from build123d import *

# Parameters (mm, degrees)
SKETCH3_R                = 50
SKETCH3_R_2              = 25
BOSS_EXTRUDE1_DEPTH      = 30
BOSS_EXTRUDE1_DEPTH_BACK = 30
SKETCH5_R                = 27.5
BOSS_EXTRUDE2_DEPTH      = 90
SKETCH6_R                = 23.5
CUT_EXTRUDE1_DEPTH       = 35
CHAMFER1_SIZE            = 1
CHAMFER3_SIZE            = 1
CHAMFER5_SIZE            = 1
CHAMFER6_SIZE            = 1
CHAMFER7_SIZE            = 1


with BuildPart() as part:
    # Sketch3 → Boss-Extrude1 (new body, two sides)
    with BuildSketch(Plane.XY) as boss_extrude1_sk:
        Circle(SKETCH3_R)
        Circle(SKETCH3_R_2, mode=Mode.SUBTRACT)
    extrude(amount=BOSS_EXTRUDE1_DEPTH)
    extrude(boss_extrude1_sk.sketch, amount=-BOSS_EXTRUDE1_DEPTH_BACK)

    # Sketch4 → Cut-Revolve5 (revolve, cut)
    with BuildSketch(Plane(origin=(0, 0, 0), x_dir=(0, 0, -1), z_dir=(1, 0, 0))):
        with BuildLine():
            Line((0, 32.5), (0, -32.5))
            ThreePointArc((0, -32.5), (32.5, 0), (0, 32.5))
        make_face()
    revolve(axis=Axis((0, 32.5, 0), (0, -1, 0)), mode=Mode.SUBTRACT)

    # Sketch5 → Boss-Extrude2 (add)
    with BuildSketch(Plane(origin=(125, 0, 0), x_dir=(0, 0, -1), z_dir=(1, 0, 0))):
        Circle(SKETCH5_R)
    extrude(amount=-BOSS_EXTRUDE2_DEPTH)

    # Sketch6 → Cut-Extrude1 (cut)
    with BuildSketch(Plane(origin=(125, 0, 0), x_dir=(0, 0, -1), z_dir=(1, 0, 0))):
        Circle(SKETCH6_R)
    extrude(amount=-CUT_EXTRUDE1_DEPTH, mode=Mode.SUBTRACT)

    # Chamfer1
    chamfer1_edges = [part.edges().sort_by_distance(p)[0] for p in [
        (-50, 0, -30),
    ]]
    chamfer(chamfer1_edges, length=CHAMFER1_SIZE)

    # Chamfer3
    chamfer3_edges = [part.edges().sort_by_distance(p)[0] for p in [
        (-25, 0, -30),
    ]]
    chamfer(chamfer3_edges, length=CHAMFER3_SIZE)

    # Chamfer5
    chamfer5_edges = [part.edges().sort_by_distance(p)[0] for p in [
        (-50, 0, 30),
    ]]
    chamfer(chamfer5_edges, length=CHAMFER5_SIZE)

    # Chamfer6
    chamfer6_edges = [part.edges().sort_by_distance(p)[0] for p in [
        (-25, 0, 30),
    ]]
    chamfer(chamfer6_edges, length=CHAMFER6_SIZE)

    # Chamfer7
    chamfer7_edges = [part.edges().sort_by_distance(p)[0] for p in [
        (125, 0, 27.5),
        (125, 0, 23.5),
    ]]
    chamfer(chamfer7_edges, length=CHAMFER7_SIZE)


solid = part.part
Geometry: final body of the model. Coordinates: model frame, mm. A direction names the side the tool comes from. Give positions to 0.01 mm unless a question says otherwise; leave off trailing zeros. Order: outer loops, then holes, each group sorted by start corner. A loop starts at its lowest first (then second) coordinate and runs counter-clockwise, first axis right, second up. Notation, with made-up numbers: (9, 69) -> (54, 69) arc R16 ccw to (54, 98) -> close; hole circle Ø8 at (69, 17). An arc over 180 degrees is marked (long way). Put each result on its own line as item: value.
Q1. Material intervals for L1, parallel to Y at x = 0, z = -26.5; L2, parallel to Y at x = 109.5, z = -1; L3, parallel to Y at x = 51, z = -9, sorted ascending.
Here are the results:
L1: y = -50 to -25, 25 to 50
L2: y = -27.48 to -23.48, 23.48 to 27.48
L3: y = -25.99 to 25.99
Q2. Draft query along X for faces 1 (the face through (-49.95, 2.2, 0.41)), 2 (the face through (107.2, 7.1, -22.4)), 3 (the face through (125, -23.43, -7.73)), 4 (the face through (23.846, 7.509, -24.826)). Return one class per face: released by +X, released by -X, zero draft, split by the parting line, or undercut.
Here are the results:
face 1: split by the parting line
face 2: zero draft
face 3: released by +X
face 4: undercut
Q3. Reachability of faces 5 (the face through (23.846, 7.509, 24.826)), 6 (the face through (83.455, 27.266, 3.58)) from +Z, -Z, +X, -X, +Y, -Y: full face, straight path, thin tool, end or side. Return the list, or none.
Here are the results:
face 5: +Z, -Z
face 6: +X
Q4. Section B-B, the plane x = 59.5. Return loops of the section in (y, z).
Here are the results:
outline: circle Ø55 at (0, 0)
Q5. Pin query (flat end, axial travel): pin 1 (8 mm diameter, centred on x = 42.5, z = 18, fed in from +Y); pin 2 (14 mm diameter, centred on y = 1, z = 11, fed in from +X); pin 3 (1.5 mm diameter, centred on y = -35, z = -8, fed in from -X). Return the tip coordinate at first contact, or that it passes through.
Here are the results:
pin 1: stops at y = 31.9
pin 2: stops at x = 90
pin 3: stops at x = -36.43
